Solid Edge part; units mm, degrees
sketch "Sketch1" plane through (0, 0, 0) normal (0, 0, 1) x (1, 0, 0)
  circle A0 centre (0, 0) radius 2.75
extrude "Protrusion1" add sketch "Sketch1" along normal blind 3
sketch "Sketch2" plane through (0, 0, 3) normal (0, 0, 1) x (1, 0, 0)
  circle A0 centre (0, 0) radius 1.5
extrude "Bult" add sketch "Sketch2" along normal blind 14
sketch "Sketch3" plane through (0, 0, 0) normal (0, 0, -1) x (1, 0, 0)
  line L0 (1.5, 0.866) -> (0, 1.7321)
  line L1 (0, 1.7321) -> (-1.5, 0.866)
  line L2 (-1.5, 0.866) -> (-1.5, -0.866)
  line L3 (-1.5, -0.866) -> (0, -1.7321)
  line L4 (0, -1.7321) -> (1.5, -0.866)
  line L5 (1.5, -0.866) -> (1.5, 0.866)
  dimension "D1" = 1.5
  dimension "D2" = 1.5
extrude "Försänkning_skruv" cut sketch "Sketch3" against normal blind 2.5
Could you check a few things on this model? Use its own coordinates, in mm. A direction names the side the tool comes from. Coordinates: 2 decimals unless noted, no trailing zeros. Order: outer loops, then holes, each group sorted by start corner. A loop starts at its lowest first (then second) coordinate and runs counter-clockwise, first axis right, second up. Notation, with made-up numbers: M -30,-12.75 L -10,-12.75 A16 ccw -10,7.25 Z; hole C 2,76.25 d2. An arc over 180 degrees is marked long. Use one line per item in the form item = value. Start each with the question number.
1. For pin 1 (1.5 mm diameter, centred on y = 0.5, z = 4, fed in from +X); pin 2 (1.5 mm diameter, centred on y = -1, z = 12.5, fed in from -X), each with a flat end and sliding along its axis, tell me the tip position at first contact or that it passes through.
2. Suppose I cut it at D-D on z = 7.5. Write out the boundary of the cut face in (x, y).
3. Please list where these lines run through material, in increasing order: line 1 (Z direction, x = -0.15, y = 2.5); line 2 (Y direction, x = -0.55, z = 1.5); line 3 (Z direction, x = -1.05, y = -0.4).
4. On a 3-axis mill with a long thin cutter (end or side, diameter ignored), from which of +Z, -Z, +X, -X, +Y, -Y can I reach the whole of each face in a straight line? I mean faces 4 (the cylindrical face through (-1.5, -0.07, 9.9)), 5 (the flat face through (0, 0, 2.5)), 6 (the flat face through (2, 0, 0)). Say none if no direction works.
5. Suppose I cut it at C-C on x = 2.15. Write out the boundary of the cut face in (y, z).
6. Suppose I cut it at B-B on y = 0. Write out the boundary of the cut face in (x, z).
7. Suppose I cut it at A-A on z = 1.25. Write out the boundary of the cut face in (x, y).
8. We'd pull the mould along X, two halves only. Please class faces 1 (the flat face through (1.2, -1.2, 3)), 2 (the flat face through (1.5, 0, 1)), 3 (the cylindrical face through (-0.596, 2.685, 1.479)): +X half, -X half, draft (parallel to the pull), parting line (faces both ways), or undercut.
Geometry says:
q1.pin_1 = 1.5
q1.pin_2 = -1.48
q2.outline = C 0,0 d3
q3.line_1 = 0 to 3
q3.line_2 = -2.69 to -1.41, 1.41 to 2.69
q3.line_3 = 2.5 to 17
q4.face_4 = +Z
q4.face_5 = -Z
q4.face_6 = -Z, +X, -X, +Y, -Y
q5.outline = M -1.71,0 L 1.71,0 L 1.71,3 L -1.71,3 Z
q6.outline = M -2.75,0 L -1.5,0 L -1.5,2.5 L 1.5,2.5 L 1.5,0 L 2.75,0 L 2.75,3 L 1.5,3 L 1.5,17 L -1.5,17 L -1.5,3 L -2.75,3 Z
q7.outline = C 0,0 d5.5; hole M -1.5,-0.87 L 0,-1.73 L 1.5,-0.87 L 1.5,0.87 L 0,1.73 L -1.5,0.87 Z
q8.face_1 = draft
q8.face_2 = undercut
q8.face_3 = parting line
